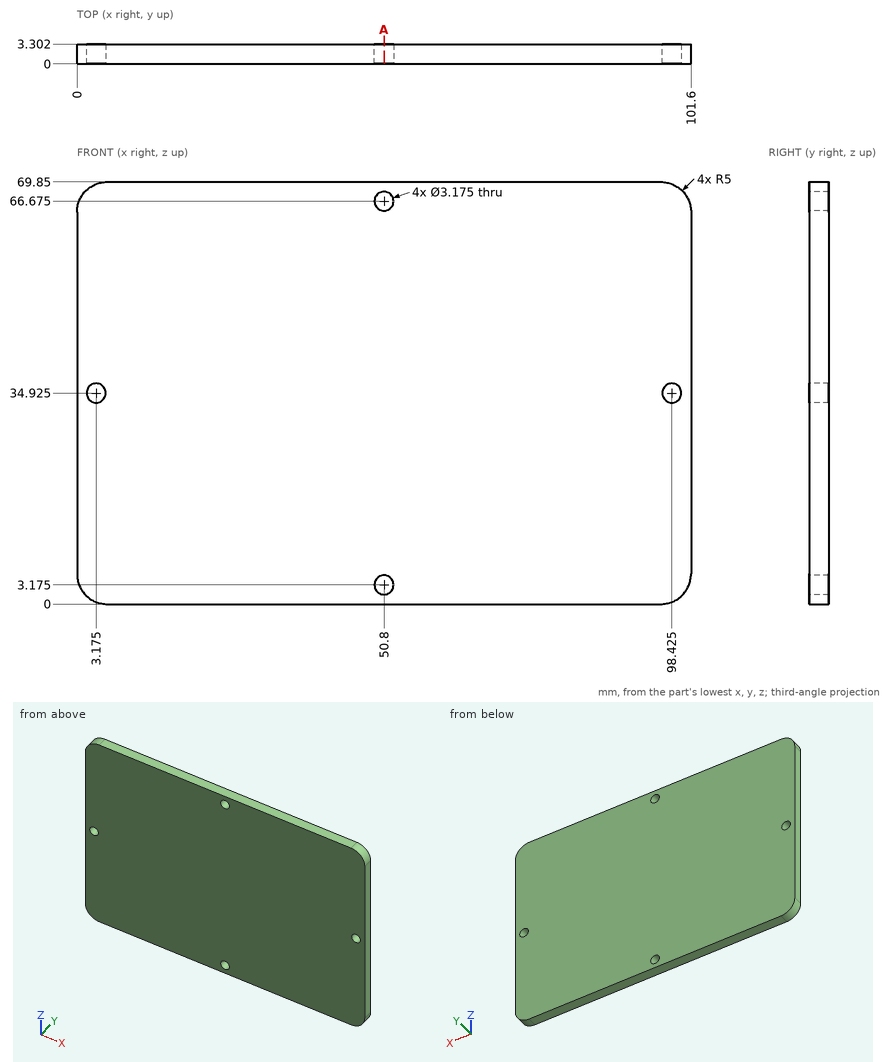
Geometry check sheet. Reference: drawing and pictorial views, mm from the part's lowest x, y, z. Round coordinates to 2 decimals unless told otherwise and drop trailing zeros. Write each loop counter-clockwise with the first axis right and the second up, starting at its lowest first coordinate (ties: lowest second). Pieces come first, ordered by that corner, then holes.
1. Scan lines: L1, parallel to Z at x = 50.8, y = 2.6; L2, parallel to Z at x = 97.5, y = 1.45; L3, parallel to X at y = 2.9, z = 65.5. Record each from-to range of solid material in increasing order.
2. Section check A-A on x = 50.8. Enter the section's corners in (y, z).
3. Gauge pin test, flat end, axial feed: P1, Ø1.9, axis at x = 50.8, z = 3.175, coming from the +Y side. Record the tip position at first contact, or that the pin passes through.
Answer:
1. L1: z = 0 to 1.59, 4.76 to 65.09, 68.26 to 69.85
1. L2: z = 0.08 to 33.63, 36.22 to 69.77
1. L3: x = 0.04 to 49.73, 51.87 to 101.56
2. outline: (0, 0) - (3.3, 0) - (3.3, 1.59) - (0, 1.59) - close; (0, 4.76) - (3.3, 4.76) - (3.3, 65.09) - (0, 65.09) - close; (0, 68.26) - (3.3, 68.26) - (3.3, 69.85) - (0, 69.85) - close
3. P1: passes through
